```python
from build123d import *

# Parameters (mm, degrees)
BOX_W             = 153.8
BOX_H             = 153.8
BOX_DEPTH         = 15
BOX001_W          = 152
BOX001_H          = 152
BOX001_DEPTH      = 13
CYLINDER002_R     = 1.6
CYLINDER002_DEPTH = 10


with BuildPart() as part:
    # Box → Box (join)
    with BuildSketch(Plane(origin=(-2, 2, 0), x_dir=(1, 0, 0), z_dir=(0, 0, -1))):
        with Locations((76.9, 76.9)):
            Rectangle(BOX_W, BOX_H)
    extrude(amount=BOX_DEPTH)

    # Box001 → Box001 (cut)
    with BuildSketch(Plane(origin=(-1.1, 1.1, 0), x_dir=(1, 0, 0), z_dir=(0, 0, -1))):
        with Locations((76, 76)):
            Rectangle(BOX001_W, BOX001_H)
    extrude(amount=BOX001_DEPTH, mode=Mode.SUBTRACT)

    # Cylinder002 → Cylinder002 (cut)
    with BuildSketch(Plane(origin=(74.9, -74.9, -19.5), x_dir=(1, 0, 0), z_dir=(0, 0, 1))):
        Circle(CYLINDER002_R)
    extrude(amount=CYLINDER002_DEPTH, mode=Mode.SUBTRACT)


solid = part.part
```
Source: CAD feature listing. Evaluate the final solid. Frame: model axes, mm. A direction names the side the tool comes from. Give positions to 0.01 mm unless a question says otherwise; leave off trailing zeros. Loops run counter-clockwise (first coordinate to the right, second up) from the corner with the lowest first, then second, coordinate; pieces in that order, holes last. Notation, with made-up numbers: (85, -1.75) -> (128, -1.75) arc R5 ccw to (128, 5.25) -> close; hole circle Ø6 at (70, 8.25). An arc over 180 degrees is marked (long way). Put each result on its own line as item: value. Start each with the question number.
1) Cut plane B-B (x = 15). Return loops of the section in (y, z), then the cut area to 3 significant figures.
2) Reachability of faces 1 (the face through (-2, -74, -7)), 2 (the face through (74, -93, -13)) from +Z, -Z, +X, -X, +Y, -Y: full face, straight path, thin tool, end or side. Return the list, or none.
3) Cut plane A-A (z = -9.75). Return loops of the section in (x, y), then the cut area to 3 significant figures.
4) Draft query along Y for faces 3 (the face through (150.9, -74, -6)), 4 (the face through (57, -76, -15)), 5 (the face through (74, -151.8, -7)). Return one class per face: released by +Y, released by -Y, zero draft, split by the parting line, or undercut.
5) Material intervals for probe 1 along X at (y, z) = (-90, -12); probe 2 along X at (y, z) = (-74.9, -13.8); probe 3 along Y at (x, z) = (74.9, -13.4), sorted ascending.
6) Cut plane C-C (y = -67). Return loops of the section in (x, z), then the cut area to 3 significant figures.
7) Contact query for a flat-ended pin moving along its axis: P1, Ø6, axis at x = 22, y = -77, coming from the +Z side. Output: stop coordinate, or through.
Results are:
1. outline: (-151.8, -15) -> (2, -15) -> (2, 0) -> (1.1, 0) -> (1.1, -13) -> (-150.9, -13) -> (-150.9, 0) -> (-151.8, 0) -> close
1. area: 331 mm2
2. face 1: +Z, -Z, -X, +Y, -Y
2. face 2: +Z
3. outline: (-2, -151.8) -> (151.8, -151.8) -> (151.8, 2) -> (-2, 2) -> close; hole (-1.1, -150.9) -> (150.9, -150.9) -> (150.9, 1.1) -> (-1.1, 1.1) -> close
3. area: 550 mm2
4. face 3: undercut
4. face 4: zero draft
4. face 5: released by -Y
5. probe 1: x = -2 to -1.1, 150.9 to 151.8
5. probe 2: x = -2 to 73.3, 76.5 to 151.8
5. probe 3: y = -151.8 to -76.5, -73.3 to 2
6. outline: (-2, -15) -> (151.8, -15) -> (151.8, 0) -> (150.9, 0) -> (150.9, -13) -> (-1.1, -13) -> (-1.1, 0) -> (-2, 0) -> close
6. area: 331 mm2
7. P1: stops at z = -13
